```python
from build123d import *

# Parameters (mm, degrees)
F2_SIZE = 0.76199


# Not quite as in the source:
# - a fillet or chamfer is up to 0.001 mm smaller than in the source, because OpenCascade refuses the exact size


with BuildPart() as f1:
    # F0 (on Front) → F1 (revolve)
    with BuildSketch(Plane.XZ):
        Polygon((2.032, 0), (1.27, 0), (1.27, -13.97), (1.27, -27.94), (3.175, -27.94), (3.175, -15.24), (6.35, -15.24), (6.35, -12.7), (2.032, -12.7), align=None)
    revolve(axis=Axis((0, 0, -18.8239812851), (0, 0, -1)))

    # F2 (size 0.762 in the source; OpenCascade refuses exactly that, so slightly less here)
    f2_edges = [f1.edges().sort_by_distance(p)[0] for p in [
        (-2.032, 0, 0),
    ]]
    chamfer(f2_edges, length=F2_SIZE)


solid = f1.part
```
Here's how the part is built. I have some questions about the finished solid (model axes, mm). A direction names the side the tool comes from. Coordinates: 2 decimals unless noted, no trailing zeros. Order: outer loops, then holes, each group sorted by start corner. A loop starts at its lowest first (then second) coordinate and runs counter-clockwise, first axis right, second up. Notation, with made-up numbers: (-26.5, 85) - (-22.5, 85) arc R17 ccw to (-22.5, 98) - close; hole circle Ø11 at (-7.75, 70.25). An arc over 180 degrees is marked (long way). One line per question, with ' | ' between items. Start each with the question number.
1. Which directions (+Z, -Z, +X, -X, +Y, -Y) give clear straight access to the entire face, cutting with the end or side of a thin tool? Please do faces 4 (the cylindrical face through (-1.38, 6.2, -13.95)), 5 (the cylindrical face through (-0.44, 1.984, -6.647)), 6 (the flat face through (2, -3, -15.24)).
2. If we section it at D-D (z = -8.5): Write out the boundary of the cut face in (x, y), and give its area (3 significant figures).
3. If we mould it in two halves opening along X, with no side actions, what happens to faces 1 (the cylindrical face through (-0.69, 3.1, -21.5)), 2 (the cylindrical face through (-0.17, -1.26, -14.17)), 3 (the flat face through (-1.4, 0.7, -27.94))? For each: released by +X, released by -X, zero draft, split by the parting line, or undercut.
4. If we section it at C-C (z = -17): Write out the boundary of the cut face in (x, y) (3 decimals).
5. I'm going to push flat-ended pins straight in: pin 1 Ø5 at (x, z) = (1.5, -22) entering from +Y (3 decimals); pin 2 Ø3 at (x, y) = (-0.5, -5) entering from +Z. Where does each tip first touch, or does it pass through?
6. Please list where these lines run through material, in increasing order: line 1 along X through (y, z) = (0, -17) (3 decimals); line 2 along Y through (x, z) = (0, -6.5). Write a range as [from, to].
Model answer:
1) face 4: +Z, -Z | face 5: +Z | face 6: -Z
2) outline: circle Ø4.06 at (0, 0); hole circle Ø2.54 at (0, 0) | area: 7.90 mm²
3) face 1: split by the parting line | face 2: undercut | face 3: zero draft
4) outline: circle Ø6.35 at (0, 0); hole circle Ø2.54 at (0, 0)
5) pin 1: stops at y = 3.175 | pin 2: stops at z = -12.7
6) line 1: x = [-3.175, -1.27], [1.27, 3.175] | line 2: y = [-2.03, -1.27], [1.27, 2.03]
